```python
from build123d import *

# Parameters (mm, degrees)
BOSS_EXTRUDE1_START         = -15
BOSS_EXTRUDE1_DEPTH         = 30
BOSS_EXTRUDE1_START_2       = -12.7
BOSS_EXTRUDE1_2_OUTLINE_W   = 10
BOSS_EXTRUDE1_2_OUTLINE_H   = 5.949524979
BOSS_EXTRUDE1_2_DEPTH       = 25.4
BOSS_EXTRUDE1_3_OUTLINE_R   = 15
BOSS_EXTRUDE1_3_OUTLINE_R_2 = 4.55
BOSS_EXTRUDE1_3_DEPTH       = 19.994560744
SKETCH4_W                   = 3.6
SKETCH4_H                   = 22.4
CUT_EXTRUDE1_DEPTH          = 6
BOSS_EXTRUDE2_REACH         = 73.536
BOSS_EXTRUDE2_END_RADIUS    = 119.634966004
SKETCH9_R                   = 6.57997386
SKETCH9_R_2                 = 3.45
SKETCH10_W                  = 5.949524979
SKETCH10_H                  = 2.3
BOSS_EXTRUDE3_DEPTH         = 10
SKETCH11_W                  = 5.949524979
SKETCH11_H                  = 30
BOSS_EXTRUDE4_DEPTH         = 10
SKETCH13_W                  = 3.6
SKETCH13_H                  = 22.4
CUT_EXTRUDE2_DEPTH          = 10
SKETCH15_R                  = 6
CUT_EXTRUDE3_DEPTH          = 5


with BuildPart() as part:
    # Boss-Extrude1: read off the stored shape, not the designer's step
    # Boss-Extrude1 outline → Boss-Extrude1 (new body)
    with BuildSketch(Plane(origin=(0, 0, 0), x_dir=(1, 0, 0), z_dir=(0, 1, 0)).offset(BOSS_EXTRUDE1_START)):
        with BuildLine():
            Line((-50, -30), (-50, -35.949524979))
            ThreePointArc((-50, -35.949524979), (-25.592440765, -27.769436157), (0, -25))
            ThreePointArc((0, -25), (25.592440765, -27.769436157), (50, -35.949524979))
            Line((50, -35.949524979), (50, -30))
            ThreePointArc((50, -30), (27.810549479, -22.327809439), (4.550000287, -19.13702996))
            ThreePointArc((4.550000287, -19.13702996), (2.275411741, -19.072115713), (0, -19.050475021))
            ThreePointArc((0, -19.050475021), (-25.592440765, -21.819911178), (-50, -30))
        make_face()
    extrude(amount=BOSS_EXTRUDE1_DEPTH)

    # Boss-Extrude1 2 outline → Boss-Extrude1 2 (add)
    with BuildSketch(Plane(origin=(0, 0, 0), x_dir=(1, 0, 0), z_dir=(0, 1, 0)).offset(BOSS_EXTRUDE1_START_2)):
        with Locations((-55, -32.97476249)):
            Rectangle(BOSS_EXTRUDE1_2_OUTLINE_W, BOSS_EXTRUDE1_2_OUTLINE_H)
    extrude(amount=BOSS_EXTRUDE1_2_DEPTH)

    # Boss-Extrude1 3 outline → Boss-Extrude1 3 (add)
    with BuildSketch(Plane.XY):
        Circle(BOSS_EXTRUDE1_3_OUTLINE_R)
        Circle(BOSS_EXTRUDE1_3_OUTLINE_R_2, mode=Mode.SUBTRACT)
    extrude(amount=BOSS_EXTRUDE1_3_DEPTH)

    # Sketch4 → Cut-Extrude1 (cut)
    with BuildSketch(Plane.XY.offset(35.949524979)):
        with Locations((-53, 0)):
            Rectangle(SKETCH4_W, SKETCH4_H)
    extrude(amount=-CUT_EXTRUDE1_DEPTH, mode=Mode.SUBTRACT)

    # Boss-Extrude2: up to this cylinder (the profile starts outside it)
    boss_extrude2_end = Plane(origin=(0, 0, 138.685441025), z_dir=(0, -1, 0)) * Cylinder(BOSS_EXTRUDE2_END_RADIUS, 387.341932008, mode=Mode.PRIVATE)
    # Sketch9 → Boss-Extrude2 (add, up to the surface)
    with BuildSketch(Plane(origin=(0, 0, 0), x_dir=(-1, 0, 0), z_dir=(0, 0, -1)), mode=Mode.PRIVATE) as boss_extrude2_sk1:
        Circle(SKETCH9_R)
        Circle(SKETCH9_R_2, mode=Mode.SUBTRACT)
    boss_extrude2_tool1 = extrude(boss_extrude2_sk1.sketch, amount=-BOSS_EXTRUDE2_REACH, mode=Mode.PRIVATE) - boss_extrude2_end
    add(boss_extrude2_tool1.solids().sort_by_distance((6.393864, 0, 0))[0])

    # Sketch10 → Boss-Extrude3 (add)
    with BuildSketch(Plane.ZY.offset(50)):
        with Locations((32.97476249, 13.85)):
            Rectangle(SKETCH10_W, SKETCH10_H)
        with Locations((32.97476249, -13.85)):
            Rectangle(SKETCH10_W, SKETCH10_H)
    extrude(amount=BOSS_EXTRUDE3_DEPTH)

    # Sketch11 → Boss-Extrude4 (add)
    with BuildSketch(Plane(origin=(50, 0, 0), x_dir=(0, 0, -1), z_dir=(1, 0, 0))):
        with Locations((-32.97476249, 0)):
            Rectangle(SKETCH11_W, SKETCH11_H)
    extrude(amount=BOSS_EXTRUDE4_DEPTH)

    # Sketch13 → Cut-Extrude2 (cut)
    with BuildSketch(Plane.XY.offset(35.949524979)):
        with Locations((53, 0)):
            Rectangle(SKETCH13_W, SKETCH13_H)
    extrude(amount=-CUT_EXTRUDE2_DEPTH, mode=Mode.SUBTRACT)

    # Sketch15 → Cut-Extrude3 (cut)
    with BuildSketch(Plane(origin=(0, 0, 0), x_dir=(-1, 0, 0), z_dir=(0, 0, -1))):
        Circle(SKETCH15_R)
    extrude(amount=-CUT_EXTRUDE3_DEPTH, mode=Mode.SUBTRACT)


solid = part.part
```
Check sheet for the modelled part. Datum: model origin and axes. Units: mm. A direction names the side the tool comes from. Give positions to 0.01 mm unless a question says otherwise; leave off trailing zeros. Order: outer loops, then holes, each group sorted by start corner. A loop starts at its lowest first (then second) coordinate and runs counter-clockwise, first axis right, second up. Notation, with made-up numbers: (0.25, -9.5) -> (24.25, -9.5) arc R19 cw to (24.25, 11.5) -> close; hole circle Ø4 at (84, 57). An arc over 180 degrees is marked (long way). Return JSON: item names as keys, results as strings.
1. Set-up check for faces 1 (the flat face through (56, 0, 30)), 2 (the cylindrical face through (0.45, 3.42, 11.95)), 3 (the flat face through (-56, 0, 35.95)), 4 (the flat face through (53, -11.2, 33)): record each of +Z, -Z, +X, -X, +Y, -Y from which the full face is reachable in a straight line by a thin tool's end or side.
From the geometry:
{"face 1": "-Z, +X, +Y, -Y", "face 2": "-Z", "face 3": "+Z, +X, -X, +Y, -Y", "face 4": "+Z, -Z"}
2. Cross-section at C-C, the plane z = 15. Record the cut outline in (x, y).
From the geometry:
{"outline": "circle Ø30 at (0, 0); hole circle Ø6.9 at (0, 0)"}
3. Cross-section at A-A, the plane y = 0. Record the cut outline in (x, z).
From the geometry:
{"outline": "(-60, 30) -> (-54.8, 30) -> (-54.8, 35.95) -> (-60, 35.95) -> close; (-51.2, 30) -> (-50, 30) arc R119.63 ccw to (-15, 19.99) -> (-15, 0) -> (-6, 0) -> (-6, 5) -> (-3.45, 5) -> (-3.45, 19.1) arc R119.63 ccw to (3.45, 19.1) -> (3.45, 5) -> (6, 5) -> (6, 0) -> (15, 0) -> (15, 19.99) arc R119.63 ccw to (50, 30) -> (51.2, 30) -> (51.2, 35.95) -> (50, 35.95) arc R119.63 cw to (-50, 35.95) -> (-51.2, 35.95) -> close; (54.8, 30) -> (60, 30) -> (60, 35.95) -> (54.8, 35.95) -> close"}
4. Cross-section at D-D, the plane x = 25.5. Record the cut outline in (y, z), plus the area to 3 significant figures.
From the geometry:
{"outline": "(-15, 21.8) -> (15, 21.8) -> (15, 27.75) -> (-15, 27.75) -> close", "area": "178 mm^2"}
5. Cross-section at B-B, the plane z = 34.5. Record the cut outline in (x, y).
From the geometry:
{"outline": "(-60, -15) -> (-46.72, -15) -> (-46.72, 15) -> (-60, 15) -> close; (46.72, -15) -> (60, -15) -> (60, 15) -> (46.72, 15) -> close; hole (-54.8, -11.2) -> (-51.2, -11.2) -> (-51.2, 11.2) -> (-54.8, 11.2) -> close; hole (51.2, -11.2) -> (54.8, -11.2) -> (54.8, 11.2) -> (51.2, 11.2) -> close"}
6. Material ranges on probe 1 along X at (y, z) = (0, 8.75); probe 2 along Y at (x, z) = (0, 2), recorded low to high. Write a range as [from, to].
From the geometry:
{"probe 1": "[-15, -3.45], [3.45, 15]", "probe 2": "[-15, -6], [6, 15]"}
7. Mould release check, pull along X, two halves, no side actions. Record for faces 5 (the flat face through (-56, 0, 30)), 6 (the cylindrical face through (6, 0, 2)), 7 (the flat face through (-60, 0, 33)): +X half, -X half, draft (parallel to the pull), parting line (faces both ways), or undercut.
From the geometry:
{"face 5": "draft", "face 6": "undercut", "face 7": "-X half"}
8. Go/stop test with flat-tipped pins: P1, Ø12, axis at x = 26, y = 1, coming from the +Z side; P2, Ø7, axis at x = 0, y = 0, coming from the -Z side; P3, Ø8, axis at y = -5, z = 14.5, coming from the +X side. Record where each tip stops, or that it passes through.
From the geometry:
{"P1": "z = 29.36", "P2": "z = 5", "P3": "x = 14.97"}
